```python
from build123d import *

# Parameters (mm, degrees)
AUSFR_SUNG_DEPTH   = 21
KREISMUSTER1_COUNT = 3


with BuildPart() as part:
    # Skizze1 → Grundk_rper (revolve)
    with BuildSketch(Plane(origin=(0, 0, 0), x_dir=(0, 0, -1), z_dir=(1, 0, 0)), mode=Mode.PRIVATE) as grundk_rper_sk:
        Polygon((95, 0), (95, 20), (50, 20), (50, 10), (0, 10), (0, 0), align=None)
    revolve(grundk_rper_sk.sketch.rotate(Axis((0, 0, 0), (0, 0, -1)), 90), axis=Axis((0, 0, 0), (0, 0, -1)))  # turned: the seam where the file's is

    # Skizze2 → Ausfr_sung (cut, through all)
    with BuildSketch(Plane(origin=(0, 0, 0), x_dir=(0, 0, -1), z_dir=(1, 0, 0))):
        with BuildLine():
            Line((100, 3), (69.866068747, 3))
            ThreePointArc((69.866068747, 3), (59.25946703, 7.393398282), (54.866068747, 18))
            Line((54.866068747, 18), (54.866068747, 23))
            Line((54.866068747, 23), (100, 23))
            Line((100, 23), (100, 3))
        make_face()
    ausfr_sung = extrude(amount=AUSFR_SUNG_DEPTH, mode=Mode.SUBTRACT)

    # Kreismuster1: Ausfr_sung ×3 about axis
    kreismuster1_axis = Axis((0, 0, 0), (0, 0, 1))
    for i in range(1, KREISMUSTER1_COUNT):
        add(ausfr_sung.rotate(kreismuster1_axis, i * 360 / KREISMUSTER1_COUNT), mode=Mode.SUBTRACT)


solid = part.part
```
Geometry check sheet. Reference: the model listing, model coordinates, mm. A direction names the side the tool comes from. Round coordinates to 2 decimals unless told otherwise and drop trailing zeros. Order: outer loops, then holes, each group sorted by start corner. A loop starts at its lowest first (then second) coordinate and runs counter-clockwise, first axis right, second up. Notation, with made-up numbers: (23.5, 53.25) - (64.5, 53.25) arc R25 ccw to (64.5, 68.25) - close; hole circle Ø4 at (70.5, -35.5). An arc over 180 degrees is marked (long way). Use a Markdown table: item, result. Add a question column.
1) Section check C-C (z = -57). Record the cut outline in (x, y), then the cut area to 3 significant figures.
2) Section check A-A (z = -14.5). Record the cut outline in (x, y).
3) Mould release check, pull along Y, two halves, no side actions. Record for faces 4 (the cylindrical face through (-10, 0, -25)), 5 (the cylindrical face through (-11.177, 4.804, -59.377)), 6 (the flat face through (15, -12, -54.866)), 7 (the flat face through (-10.06, -5.81, -75.21)): released by +Y, released by -Y, zero draft, split by the parting line, or undercut.
4) Gauge pin test, flat ends, axial feed: P1, Ø2, axis at x = 0, z = -81, coming from the -Y side; P2, Ø1.5, axis at x = -12, y = -1.5, coming from the -Z side; P3, Ø8.5, axis at y = 11, z = -76.5, coming from the +X side. Record the tip position at first contact, or that the pin passes through.
5) Set-up check for faces 1 (the flat face through (3, 19, -54.866)), 2 (the flat face through (-5, -9, -50)), 3 (the flat face through (-18, -6, -54.866)): record each of +Z, -Z, +X, -X, +Y, -Y from which the full face is reachable in a straight line by a thin tool's end or side.
6) Thickness scan on line 1 along Z through (x, y) = (15, -6.5); line 2 along Y through (x, z) = (-3.5, -75); line 3 along Y through (x, z) = (14, -52). Record the ranges inside material, lowest first.
7) Section check B-B (z = -68). Record the cut outline in (x, y).
Established:
| question | item | result |
|---|---|---|
| 1 | outline | (-17.49, 9.71) - (-8.91, -5.14) - (-17.32, -10) arc R20 ccw to (0.33, -20) - (8.91, -5.14) - (17.32, -10) arc R20 ccw to (17.15, 10.29) - (0, 10.29) - (0, 20) arc R20 ccw to start |
| 1 | area | 903 mm2 |
| 2 | outline | circle Ø20 at (0, 0) |
| 3 | face 4 | split by the parting line |
| 3 | face 5 | undercut |
| 3 | face 6 | zero draft |
| 3 | face 7 | undercut |
| 4 | P1 | y = -7.73 |
| 4 | P2 | z = -56.94 |
| 4 | P3 | x = 0 |
| 5 | face 1 | -Z, +X, +Y |
| 5 | face 2 | +Z |
| 5 | face 3 | -Z, -X |
| 6 | line 1 | -95 to -50 |
| 6 | line 2 | -12.06 to -2.02, 0.06 to 19.69 |
| 6 | line 3 | -14.28 to 14.28 |
| 7 | outline | (-17.32, -10) arc R20 ccw to (-7.18, -18.67) - (2.7, -1.56) - (17.32, -10) arc R20 ccw to (19.76, 3.12) - (0, 3.12) - (0, 20) arc R20 ccw to (-12.58, 15.55) - (-2.7, -1.56) - close |
